from build123d import *

# Parameters (mm, degrees)
SKETCH1_W               = 315
SKETCH1_H               = 54
BOSS_EXTRUDE2_DEPTH     = 60
CUT_EXTRUDE2_DEPTH      = 25
CUT_EXTRUDE2_DEPTH_BACK = 25
BOSS_EXTRUDE3_DEPTH     = 1
SKETCH9_W               = 48
SKETCH9_H               = 50
CUT_EXTRUDE5_DEPTH      = 167.012800738
SKETCH10_R              = 12
CUT_EXTRUDE6_DEPTH      = 2
SKETCH11_R              = 1.65
CUT_EXTRUDE7_DEPTH      = 177.98093121
CUT_EXTRUDE8_DEPTH      = 2.3
CUT_EXTRUDE9_DEPTH      = 2.3


with BuildPart() as part:
    # Sketch1 → Boss-Extrude2 (new body)
    with BuildSketch(Plane(origin=(0, 0, 0), x_dir=(1, 0, 0), z_dir=(0, 1, 0))):
        Rectangle(SKETCH1_W, SKETCH1_H)
    extrude(amount=BOSS_EXTRUDE2_DEPTH)

    # Sketch7 → Cut-Extrude2 (cut, two sides: drawn at the far end of the back side and taken through both)
    with BuildSketch(Plane.XY.offset(-CUT_EXTRUDE2_DEPTH_BACK)):
        with BuildLine():
            Line((-141.5, 33.764258555), (-24, 15))
            Line((-24, 15), (24, 15))
            Line((24, 15), (141.5, 33.764258555))
            add(Edge.make_bspline(
                [(141.5, 33.764258555), (155.5, 36), (155.5, 60)],
                knots=[3.234883811, 3.234883811, 3.234883811, 4.71238898, 4.71238898, 4.71238898], degree=2, weights=[1, 0.739309101, 1]))
            Line((155.5, 60), (-155.5, 60))
            add(Edge.make_bspline(
                [(-155.5, 60), (-155.5, 36), (-141.5, 33.764258555)],
                knots=[4.71238898, 4.71238898, 4.71238898, 6.18989415, 6.18989415, 6.18989415], degree=2, weights=[1, 0.739309101, 1]))
        make_face()
    extrude(amount=CUT_EXTRUDE2_DEPTH + CUT_EXTRUDE2_DEPTH_BACK, mode=Mode.SUBTRACT)

    # Sketch7<2> → Boss-Extrude3 (add, symmetric)
    with BuildSketch(Plane.XY):
        with BuildLine():
            Line((-141.5, 33.764258555), (-24, 15))
            Line((-24, 15), (24, 15))
            Line((24, 15), (141.5, 33.764258555))
            add(Edge.make_bspline(
                [(141.5, 33.764258555), (155.5, 36), (155.5, 60)],
                knots=[3.234883811, 3.234883811, 3.234883811, 4.71238898, 4.71238898, 4.71238898], degree=2, weights=[1, 0.739309101, 1]))
            Line((155.5, 60), (-155.5, 60))
            add(Edge.make_bspline(
                [(-155.5, 60), (-155.5, 36), (-141.5, 33.764258555)],
                knots=[4.71238898, 4.71238898, 4.71238898, 6.18989415, 6.18989415, 6.18989415], degree=2, weights=[1, 0.739309101, 1]))
        make_face()
    extrude(amount=BOSS_EXTRUDE3_DEPTH, both=True)

    # Sketch9 → Cut-Extrude5 (cut, through all)
    with BuildSketch(Plane(origin=(0, 15, 0), x_dir=(1, 0, 0), z_dir=(0, 1, 0))):
        Rectangle(SKETCH9_W, SKETCH9_H)
    extrude(amount=CUT_EXTRUDE5_DEPTH, mode=Mode.SUBTRACT)

    # Sketch10 → Cut-Extrude6 (cut)
    with BuildSketch(Plane.XZ):
        with Locations(Location((0, 0, 0), (0, 0, 270))):
            Circle(SKETCH10_R)
    extrude(amount=-CUT_EXTRUDE6_DEPTH, mode=Mode.SUBTRACT)

    # Sketch4 for Cut-Loft3 → Cut-Loft3 section 0
    with BuildSketch(Plane.XZ.offset(-2)):
        with BuildLine():
            # circular arc as an exact rational Bezier (weights 1, cos(half-angle), 1)
            Bezier((-8.310381938, 8.656647852), (0, 16.634614514), (8.310381938, 8.656647852), weights=[1, 0.721387321, 1])
            Bezier((8.310381938, 8.656647852), (17.327723452, 0), (8.310381938, -8.656647852), weights=[1, 0.692531828, 1])
            Bezier((8.310381938, -8.656647852), (0, -16.634614514), (-8.310381938, -8.656647852), weights=[1, 0.721387321, 1])
            Bezier((-8.310381938, -8.656647852), (-17.327723452, 0), (-8.310381938, 8.656647852), weights=[1, 0.692531828, 1])
        make_face()
    # Sketch9<2> → Cut-Loft3 section 1
    with BuildSketch(Plane(origin=(0, 15, 0), x_dir=(1, 0, 0), z_dir=(0, 1, 0))):
        with BuildLine():
            Line((-24, -25), (24, -25))
            Line((24, -25), (24, 25))
            Line((24, 25), (-24, 25))
            Line((-24, 25), (-24, -25))
        make_face()
    loft(mode=Mode.SUBTRACT)

    # Sketch11 → Cut-Extrude7 (cut, through all)
    with BuildSketch(Plane.XY.offset(27)):
        with Locations((-152.5, 35)):
            Circle(SKETCH11_R)
        with Locations((152.5, 35)):
            Circle(SKETCH11_R)
        Polygon((-157.5, 31.091711648), (-14, 0), (-157.5, 0), align=None)
        Polygon((157.5, 31.091711648), (157.5, 0), (14, 0), align=None)
        Polygon((-118.160810021, 60), (-119.042024296, 54.481920135), (-24, 39.304106369), (-23.118785725, 44.822186234), (0, 41.130212848), (23.118785725, 44.822186234), (24, 39.304106369), (119.042024296, 54.481920135), (118.160810021, 60), align=None)
    extrude(amount=-CUT_EXTRUDE7_DEPTH, mode=Mode.SUBTRACT)

    # Sketch12 → Cut-Extrude8 (cut)
    with BuildSketch(Plane.XY.offset(19)):
        Polygon((-150.854551733, 37.85), (-157.5, 37.85), (-157.5, 32.15), (-150.854551733, 32.15), (-149.209103466, 35), align=None)
        Polygon((157.5, 37.85), (157.5, 32.15), (150.854551733, 32.15), (149.209103466, 35), (150.854551733, 37.85), align=None)
    extrude(amount=-CUT_EXTRUDE8_DEPTH, mode=Mode.SUBTRACT)

    # Sketch13 → Cut-Extrude9 (cut)
    with BuildSketch(Plane(origin=(0, 0, -19), x_dir=(-1, 0, 0), z_dir=(0, 0, -1))):
        Polygon((-150.854551733, 37.85), (-157.5, 37.85), (-157.5, 32.15), (-150.854551733, 32.15), (-149.209103466, 35), align=None)
        Polygon((157.5, 37.85), (157.5, 32.15), (150.854551733, 32.15), (149.209103466, 35), (150.854551733, 37.85), align=None)
    extrude(amount=-CUT_EXTRUDE9_DEPTH, mode=Mode.SUBTRACT)


solid = part.part
Input: part model. Units: mm. Frame: model coordinates. A direction names the side the tool comes from. Give positions to 0.01 mm unless a question says otherwise; leave off trailing zeros. Write each loop counter-clockwise with the first axis right and the second up, starting at its lowest first coordinate (ties: lowest second). Pieces come first, ordered by that corner, then holes. Notation, with made-up numbers: (-38.75, -6.5) -> (4.25, -6.5) arc R32 ccw to (4.25, 32.5) -> close; hole circle Ø6 at (14.25, 19.25). An arc over 180 degrees is marked (long way). Use one line per item in the form item = value. Start each with the question number.
1) Ray query, probe 1 along Z at (x, y) = (-143.5, 38); probe 2 along X at (y, z) = (34.5, 7); probe 3 along Z at (x, y) = (11, 40.5). Return the intervals inside material, ascending. Write a range as from..to.
2) Set-up query: faces 4 (the flat face through (-154.3, 35, -16.7)), 5 (the flat face through (-2, 30, -27)), 6 (the flat face through (-91, 38, -1)). Return all of +Z, -Z, +X, -X, +Y, -Y with unobstructed straight access to the full face (end or side cutting, diameter ignored); none if empty.
3) Section query A-A on x = -85. Return the cut outline in (y, z), then the cut area to 3 significant figures.
4) Pin query (flat end, axial travel): pin 1 (12 mm diameter, centred on x = 40.5, z = -21.5, fed in from -Y); pin 2 (12 mm diameter, centred on x = 21, z = 7.5, fed in from -Y); pin 3 (4 mm diameter, centred on x = 125.5, z = 3.5, fed in from -Y). Return the tip coordinate at first contact, or that it passes through.
5) Draft query along Y for faces 1 (the flat face through (154.3, 35, 16.7)), 2 (the flat face through (142, 60, 0)), 3 (the flat face through (157.5, 45, 0)). Return one class per face: pulls with the +Y half, pulls with the -Y half, needs draft (parallel to the pull), parting line crosses it, or undercut.
6) Section query B-B on x = 51.5. Return the cut outline in (y, z), then the cut area to 3 significant figures.
Outcome:
q1.probe_1 = -27..-25, -1..1, 25..27
q1.probe_2 = -157.5..-154.07, -150.93..-143.95, 143.95..150.93, 154.07..157.5
q1.probe_3 = -27..-25, 25..27
q2.face_4 = -X
q2.face_5 = -Z, +X, -X, +Y, -Y
q2.face_6 = +Y
q3.outline = (15.38, -27) -> (49.05, -27) -> (49.05, -25) -> (24.74, -25) -> (24.74, -1) -> (49.05, -1) -> (49.05, 1) -> (24.74, 1) -> (24.74, 25) -> (49.05, 25) -> (49.05, 27) -> (15.38, 27) -> close
q3.area = 651 mm^2
q4.pin_1 = 4.44
q4.pin_2 = 0.22
q4.pin_3 = 23.73
q5.face_1 = undercut
q5.face_2 = pulls with the +Y half
q5.face_3 = needs draft
q6.outline = (8.13, -27) -> (43.7, -27) -> (43.7, -25) -> (19.39, -25) -> (19.39, -1) -> (43.7, -1) -> (43.7, 1) -> (19.39, 1) -> (19.39, 25) -> (43.7, 25) -> (43.7, 27) -> (8.13, 27) -> close
q6.area = 754 mm^2
